from build123d import *

# Parameters (mm, degrees)
SKETCH2_R          = 7.5
CUT_EXTRUDE1_DEPTH = 35


with BuildPart() as part:
    # Sketch1 → Revolve1 (revolve)
    with BuildSketch(Plane.XY, mode=Mode.PRIVATE) as revolve1_sk:
        Polygon((20, 0), (20, 80), (30, 80), (30, 50), (35, 10), (40, 10), (40, 0), align=None)
    revolve(revolve1_sk.sketch.rotate(Axis((0, 0, 0), (0, 1, 0)), 90), axis=Axis((0, 0, 0), (0, 1, 0)))

    # Sketch2 → Cut-Extrude1 (cut, symmetric)
    with BuildSketch(Plane.XY):
        with Locations((0, 65)):
            Circle(SKETCH2_R)
    extrude(amount=CUT_EXTRUDE1_DEPTH, both=True, mode=Mode.SUBTRACT)


solid = part.part
Part model, mm, in its own coordinate system. A direction names the side the tool comes from. Give positions to 0.01 mm unless a question says otherwise; leave off trailing zeros. Write each loop counter-clockwise with the first axis right and the second up, starting at its lowest first coordinate (ties: lowest second). Pieces come first, ordered by that corner, then holes.
1) Cut at C-C on y = 59.5. Write the cut outline in (x, z), then the cut area to 3 significant figures.
Resolved:
outline: (-5.1, -29.56) - (-5.1, -19.34) arc R20 cw to (-5.1, 19.34) - (-5.1, 29.56) arc R30 ccw to start; (5.1, -29.56) arc R30 ccw to (5.1, 29.56) - (5.1, 19.34) arc R20 cw to (5.1, -19.34) - close
area: 1,370 mm2
2) Two-plate mould, pull along X, no slides. Class faces 3 (the face through (35.4, 10, -0.2)), 4 (the face through (-1.76, 4.93, 39.96)), 5 (the face through (-5.5, 70.1, 24.4)): released by +X, released by -X, zero draft, split by the parting line, or undercut.
Resolved:
face 3: zero draft
face 4: split by the parting line
face 5: undercut
3) Probe L1, parallel to Y at x = 0, z = 24.25; L2, parallel to X at y = 24, z = -18.5; L3, parallel to Z at x = -18, y = 55. List the from-to ranges inside material, lowest first.
Resolved:
L1: y = 0 to 57.5, 72.5 to 80
L2: x = -27.63 to -7.6, 7.6 to 27.63
L3: z = -24 to -8.72, 8.72 to 24
4) Cut at D-D on y = 28. Write the cut outline in (x, z).
Resolved:
outline: circle Ø65.5 at (0, 0); hole circle Ø40 at (0, 0)
5) Cut at B-B on x = 0. Write the cut outline in (y, z).
Resolved:
outline: (0, -40) - (10, -40) - (10, -35) - (50, -30) - (57.5, -30) - (57.5, -20) - (0, -20) - close; (0, 20) - (57.5, 20) - (57.5, 30) - (50, 30) - (10, 35) - (10, 40) - (0, 40) - close; (72.5, -30) - (80, -30) - (80, -20) - (72.5, -20) - close; (72.5, 20) - (80, 20) - (80, 30) - (72.5, 30) - close
6) Cut at A-A on z = 0. Write the cut outline in (x, y).
Resolved:
outline: (-40, 0) - (-20, 0) - (-20, 80) - (-30, 80) - (-30, 50) - (-35, 10) - (-40, 10) - close; (20, 0) - (40, 0) - (40, 10) - (35, 10) - (30, 50) - (30, 80) - (20, 80) - close
7) Pin check, flat tips, straight feed: pin 1 (2 mm diameter, centred on y = 57, z = -19, fed in from -X); pin 2 (6 mm diameter, centred on y = 9.5, z = 26, fed in from +X); pin 3 (9 mm diameter, centred on x = 0, y = 65, fed in from +Z); pin 4 (8 mm diameter, centred on y = 38, z = -8, fed in from +X). Stop position of each tip, or through.
Resolved:
pin 1: stops at x = -24
pin 2: stops at x = 32.73
pin 3: passes through
pin 4: stops at x = 31.44
8) Which spindle directions (+Z, -Z, +X, -X, +Y, -Y) get a long thin tool onto all of the face, cutting with end or side? Do faces 1 (the face through (-5.952, 60.436, -24.19)), 2 (the face through (-9.011, 64.79, -28.615)). Say none if no direction does.
Resolved:
face 1: +Z, -Z
face 2: +Y
